Work out the finished part from the listing and answer in its coordinate system (mm). A direction names the side the tool comes from. Round coordinates to 2 decimals unless told otherwise and drop trailing zeros. Order: outer loops, then holes, each group sorted by start corner. A loop starts at its lowest first (then second) coordinate and runs counter-clockwise, first axis right, second up. Notation, with made-up numbers: (80, 54.25) -> (133, 54.25) arc R27 cw to (133, 82.25) -> close; hole circle Ø9 at (50, -38.5). An arc over 180 degrees is marked (long way). Use a Markdown table: item, result. Add a question column.
Item 1: Flat-ended cylindrical pins translate along their axes: P1, Ø4, axis at x = -40.5, y = 23, coming from the +Z side; P2, Ø18, axis at x = 53.5, y = 86, coming from the -Z side; P3, Ø10, axis at x = 43, z = -49.5, coming from the -Y side; P4, Ø10, axis at x = -53.5, y = 98.5, coming from the +Z side. Find the tip coordinate at first contact, or state that the pin passes through.
Item 2: A cutting plane is placed at B-B, the plane y = 75. Determine the outline of the cut face in (x, z).
Item 3: A cutting plane is placed at A-A, the plane x = 0. Determine the outline of the cut face in (y, z).
Item 4: A tool of negligible diameter and unlimited length cuts with its end or side. For faces 1 (the flat face through (46, 28, 0)), 2 (the flat face through (42, 25, 16)), 3 (the flat face through (66, 270, 10)), from which of +Z, -Z, +X, -X, +Y, -Y can it reach the whole face along a straight path? Write none if from no direction.
Item 5: A cutting plane is placed at D-D, the plane y = 260. Determine the outline of the cut face in (x, z), plus the area to 3 significant figures.
Item 6: A cutting plane is placed at C-C, the plane z = -10. Determine the outline of the cut face in (x, y).
Item 7: Find the intervals of material crossed by L1, parallel to X at y = 30, z = 14; L2, parallel to Z at x = 61.5, y = 185; L3, parallel to X at y = 267, z = -34.5 (3 decimals), in increasing order. Write a range as [from, to].
from build123d import *

# Parameters (mm, degrees)
EXTRUDE_4_DEPTH     = 20
EXTRUDE_START       = 50
EXTRUDE_8_DEPTH     = 20
SKETCH_16_W         = 8
SKETCH_16_H         = 40
SKETCH_19_W         = 8
SKETCH_19_H         = 40
SKETCH_21_R         = 16
EXTRUDE_13_DEPTH    = 8
EXTRUDE_START_2     = -8
SKETCH_22_R         = 16
EXTRUDE_14_DEPTH    = 8
SKETCH_23_W         = 7.590296008
SKETCH_23_H         = 50
CUT_EXTRUDE_2_DEPTH = 323.453097365


# Read off the part's stored shape, not the designer's step: the extrude step
with BuildPart() as part:
    # Sketch 3D_1 → Extrude 4 (new, symmetric)
    with BuildSketch(Plane(origin=(-74, 270, 0), x_dir=(0.9909924304103234, 0, 0.13391789600139506), z_dir=(0, -1, 0))):
        with BuildLine():
            Line((0, 0), (2.67835792, 19.819848608))
            Line((2.67835792, 19.819848608), (10.606297363, 18.74850544))
            Line((10.606297363, 18.74850544), (7.927939443, -1.071343168))
            ThreePointArc((7.927939443, -1.071343168), (64.494858714, -75.315424711), (138.738940257, -18.74850544))
            Line((138.738940257, -18.74850544), (141.417298177, 1.071343168))
            Line((141.417298177, 1.071343168), (149.345237621, 0))
            Line((149.345237621, 0), (146.666879701, -19.819848608))
            ThreePointArc((146.666879701, -19.819848608), (63.423515546, -83.243364154), (0, 0))
        make_face()
    extrude(amount=EXTRUDE_4_DEPTH, both=True)



with BuildPart() as body_2:
    # Extrude 8 outline → Extrude 8 (new body)
    with BuildSketch(Plane(origin=(0, 0, 0), x_dir=(1, 0, 0), z_dir=(0, 1, 0)).offset(EXTRUDE_START)):
        with BuildLine():
            Line((38, 0), (38, -20))
            Line((38, -20), (46, -20))
            Line((46, -20), (46, 0))
            ThreePointArc((46, 0), (0, 46), (-46, 0))
            Line((-46, 0), (-46, -20))
            Line((-46, -20), (-38, -20))
            Line((-38, -20), (-38, 0))
            ThreePointArc((-38, 0), (0, 38), (38, 0))
        make_face()
    extrude(amount=EXTRUDE_8_DEPTH)


with BuildPart() as part_1:
    add(part.part)

    add(body_2.part)  # Sweep 5 merges body 2
    # Sweep 5: sweep along a path in Sketch 18
    with BuildLine(Plane.XY.offset(20)) as sweep_5_path:
        Line((-46, 0), (-46, 50))
        Line((-46, 50), (-46, 70))
        Line((-46, 70), (-74, 250))
        Line((-74, 250), (-74, 290))
    # Sketch 16 → Sweep 5 (sweep)
    with BuildSketch(Plane(origin=(0, 0, 0), x_dir=(1, 0, 0), z_dir=(0, 1, 0))):
        with Locations((-42, 0)):
            Rectangle(SKETCH_16_W, SKETCH_16_H)
    sweep(path=sweep_5_path.line, transition=Transition.RIGHT)

    # Sweep 6: sweep along a path in Sketch 20
    with BuildLine(Plane.XY.offset(20)) as sweep_6_path:
        Line((46, 0), (46, 50))
        Line((46, 50), (46, 70))
        Line((46, 70), (74, 250))
        Line((74, 250), (74, 290))
    # Sketch 19 → Sweep 6 (sweep)
    with BuildSketch(Plane(origin=(0, 0, 0), x_dir=(1, 0, 0), z_dir=(0, 1, 0))):
        with Locations((42, 0)):
            Rectangle(SKETCH_19_W, SKETCH_19_H)
    sweep(path=sweep_6_path.line, transition=Transition.RIGHT)

    # Sketch 21 → Extrude 13 (add)
    with BuildSketch(Plane(origin=(46, 0, 0), x_dir=(0, 0, -1), z_dir=(1, 0, 0))):
        Circle(SKETCH_21_R)
    extrude(amount=-EXTRUDE_13_DEPTH)

    # Sketch 22 → Extrude 14 (add)
    with BuildSketch(Plane.ZY.offset(46).offset(EXTRUDE_START_2)):
        Circle(SKETCH_22_R)
    extrude(amount=EXTRUDE_14_DEPTH)

    # Sketch 23 → Cut-Extrude 2 (cut, through all)
    with BuildSketch(Plane.ZY.offset(46)):
        with Locations((19.795148004, 25)):
            Rectangle(SKETCH_23_W, SKETCH_23_H)
    extrude(amount=-CUT_EXTRUDE_2_DEPTH, mode=Mode.SUBTRACT)


solid = part_1.part
Reported:
| question | item | result |
|---|---|---|
| 1 | P1 | z = 16 |
| 1 | P2 | z = -20 |
| 1 | P3 | y = 250 |
| 1 | P4 | z = 20 |
| 2 | outline | (-46.78, -20) -> (-38.68, -20) -> (-38.68, 20) -> (-46.78, 20) -> close; (38.68, -20) -> (46.78, -20) -> (46.78, 20) -> (38.68, 20) -> close |
| 3 | outline | (50, -46) -> (70, -46) -> (70, -38) -> (50, -38) -> close; (250, -74) -> (290, -74) -> (290, -66) -> (250, -66) -> close |
| 4 | face 1 | +Z, -Z, +X, -Y |
| 4 | face 2 | +Z, +X, -X, -Y |
| 4 | face 3 | +Z, +Y |
| 5 | outline | (-74, -20) -> (-71.25, -20) arc R74 ccw to (71.25, -20) -> (74, -20) -> (74, 20) -> (66, 20) -> (66, 0) arc R66 cw to (-66, 0) -> (-66, 20) -> (-74, 20) -> close |
| 5 | area | 2,120 mm² |
| 6 | outline | (-74, 250) -> (-46, 70) -> (-46, -12.49) -> (-38, -12.49) -> (-38, 50) -> (-36.66, 50) -> (-36.66, 70) -> (-38, 70) -> (-38, 70.62) -> (-65.9, 250) -> (-65.24, 250) -> (-65.24, 290) -> (-74, 290) -> close; (36.66, 50) -> (38, 50) -> (38, -12.49) -> (46, -12.49) -> (46, 70) -> (74, 250) -> (74, 290) -> (65.24, 290) -> (65.24, 250) -> (65.9, 250) -> (38, 70.62) -> (38, 70) -> (36.66, 70) -> close |
| 7 | L1 | [-46, -38], [38, 46] |
| 7 | L2 | [-20, 20] |
| 7 | L3 | [-65.466, -56.265], [56.265, 65.466] |
